Geometry check sheet. Reference: the model listing, model coordinates, mm. Face numbers are marked on the shaded views. A direction names the side the tool comes from. Coordinates: 2 decimals unless noted, no trailing zeros. Write each loop counter-clockwise with the first axis right and the second up, starting at its lowest first coordinate (ties: lowest second). Pieces come first, ordered by that corner, then holes. Notation, with made-up numbers: (59, 48) -> (67, 48) arc R15 cw to (67, 61) -> close; hole circle Ø5 at (52, 38.25). An arc over 180 degrees is marked (long way). Use a Markdown table: item, result.
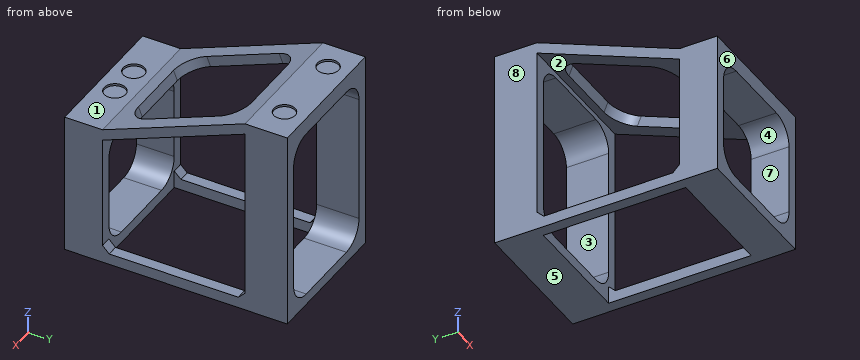
```python
from build123d import *

# Parameters (mm, degrees)
BOSS_EXTRUDE1_DEPTH = 58.71
SKETCH4_R           = 4.8
CUT_EXTRUDE1_DEPTH  = 1
SKETCH5_R           = 4.8
CUT_EXTRUDE2_DEPTH  = 1
SKETCH6_W           = 19
SKETCH6_H           = 26
BOSS_EXTRUDE3_DEPTH = 58.71
SKETCH7_W           = 58.71
SKETCH7_H           = 17
SKETCH7_H_2         = 19
BOSS_EXTRUDE4_DEPTH = 59
BOSS_EXTRUDE5_DEPTH = 3
CUT_EXTRUDE3_DEPTH  = 17
CUT_EXTRUDE4_START  = -19
CUT_EXTRUDE4_DEPTH  = 19
CUT_EXTRUDE5_DEPTH  = 4.632332886
SKETCH12_W          = 5
SKETCH12_H          = 5
BOSS_EXTRUDE6_DEPTH = 100
CHAMFER1_SIZE       = 3


with BuildPart() as part:
    # Sketch3 → Boss-Extrude1 (new body)
    with BuildSketch(Plane.YZ):
        Polygon((0, 5), (0, 0), (17, 0), (81, 26), (100, 26), (100, 31), (81, 31), (17, 5), align=None)
    extrude(amount=BOSS_EXTRUDE1_DEPTH)

    # Sketch4 → Cut-Extrude1 (cut)
    with BuildSketch(Plane.XY.offset(31)):
        with Locations((12.75, 90.5)):
            Circle(SKETCH4_R)
        with Locations((47.2, 90.5)):
            Circle(SKETCH4_R)
    extrude(amount=-CUT_EXTRUDE1_DEPTH, mode=Mode.SUBTRACT)

    # Sketch5 → Cut-Extrude2 (cut)
    with BuildSketch(Plane.XY.offset(5)):
        with Locations((21.94, 8.5)):
            Circle(SKETCH5_R)
        with Locations((36.94, 8.5)):
            Circle(SKETCH5_R)
    extrude(amount=-CUT_EXTRUDE2_DEPTH, mode=Mode.SUBTRACT)

    # Sketch6 → Boss-Extrude3 (add)
    with BuildSketch(Plane.YZ.offset(58.71)):
        with Locations((90.5, 13)):
            Rectangle(SKETCH6_W, SKETCH6_H)
    extrude(amount=-BOSS_EXTRUDE3_DEPTH)

    # Sketch7 → Boss-Extrude4 (add)
    with BuildSketch(Plane(origin=(0, 0, 0), x_dir=(1, 0, 0), z_dir=(0, 0, -1))):
        with Locations((29.355, -8.5)):
            Rectangle(SKETCH7_W, SKETCH7_H)
        with Locations((29.355, -90.5)):
            Rectangle(SKETCH7_W, SKETCH7_H_2)
    extrude(amount=BOSS_EXTRUDE4_DEPTH)

    # Sketch8 → Boss-Extrude5 (add)
    with BuildSketch(Plane.YZ.offset(58.71)):
        Polygon((100, 31), (81, 31), (17, 5), (0, 5), (0, -59), (17, -59), (17, 0), (81, 26), (81, -59), (100, -59), align=None)
    extrude(amount=BOSS_EXTRUDE5_DEPTH)

    # Sketch9 → Cut-Extrude3 (cut)
    with BuildSketch(Plane.XZ):
        with BuildLine():
            Line((15, -2.5), (46.71, -2.5))
            ThreePointArc((46.71, -2.5), (53.781067812, -5.428932188), (56.71, -12.5))
            Line((56.71, -12.5), (56.71, -44))
            ThreePointArc((56.71, -44), (53.781067812, -51.071067812), (46.71, -54))
            Line((46.71, -54), (15, -54))
            ThreePointArc((15, -54), (7.928932188, -51.071067812), (5, -44))
            Line((5, -44), (5, -12.5))
            ThreePointArc((5, -12.5), (7.928932188, -5.428932188), (15, -2.5))
        make_face()
    extrude(amount=-CUT_EXTRUDE3_DEPTH, mode=Mode.SUBTRACT)

    # Sketch10 → Cut-Extrude4 (cut)
    with BuildSketch(Plane(origin=(0, 100, 0), x_dir=(-1, 0, 0), z_dir=(0, 1, 0)).offset(CUT_EXTRUDE4_START)):
        with BuildLine():
            Line((-46.71, 23.5), (-15, 23.5))
            ThreePointArc((-15, 23.5), (-7.928932188, 20.571067812), (-5, 13.5))
            Line((-5, 13.5), (-5, -44))
            ThreePointArc((-5, -44), (-7.928932188, -51.071067812), (-15, -54))
            Line((-15, -54), (-46.71, -54))
            ThreePointArc((-46.71, -54), (-53.781067812, -51.071067812), (-56.71, -44))
            Line((-56.71, -44), (-56.71, 13.5))
            ThreePointArc((-56.71, 13.5), (-53.781067812, 20.571067812), (-46.71, 23.5))
        make_face()
    extrude(amount=CUT_EXTRUDE4_DEPTH, mode=Mode.SUBTRACT)

    # Sketch11 → Cut-Extrude5 (cut)
    with BuildSketch(Plane(origin=(0, 0.664710813, -1.636211232), x_dir=(1, 0, 0), z_dir=(0, -0.376377046955938, 0.9264665771223093))):
        with BuildLine():
            Line((17, 79.711481203), (44.71, 79.711481203))
            ThreePointArc((44.71, 79.711481203), (51.781067812, 76.782549014), (54.71, 69.711481203))
            Line((54.71, 69.711481203), (54.71, 34.631817046))
            ThreePointArc((54.71, 34.631817046), (51.781067812, 27.560749234), (44.71, 24.631817046))
            Line((44.71, 24.631817046), (17, 24.631817046))
            ThreePointArc((17, 24.631817046), (9.928932188, 27.560749234), (7, 34.631817046))
            Line((7, 34.631817046), (7, 69.711481203))
            ThreePointArc((7, 69.711481203), (9.928932188, 76.782549014), (17, 79.711481203))
        make_face()
    extrude(amount=-CUT_EXTRUDE5_DEPTH, mode=Mode.SUBTRACT)

    # Sketch12 → Boss-Extrude6 (add)
    with BuildSketch(Plane.XZ):
        with Locations((2.5, -56.5)):
            Rectangle(SKETCH12_W, SKETCH12_H)
        with Locations((59.21, -56.5)):
            Rectangle(SKETCH12_W, SKETCH12_H)
    extrude(amount=-BOSS_EXTRUDE6_DEPTH)

    # Chamfer1
    chamfer1_edges = [part.edges().sort_by_distance(p)[0] for p in [
        (2.5, 17, -54),
        (2.5, 81, -54),
        (59.21, 81, -54),
        (59.21, 17, -54),
    ]]
    chamfer(chamfer1_edges, length=CHAMFER1_SIZE)


solid = part.part
```
Item 1: Depth check by flat-ended pin: P1, Ø12, axis at x = 27.5, y = 19, coming from the +Z side; P2, Ø13.5, axis at x = 37.5, y = 5, coming from the +Z side; P3, Ø3, axis at x = 7, y = 56, coming from the -Z side. Enter the tip coordinate at first touch or a pass-through.
Answer block:
| item | result |
|---|---|
| P1 | stops at z = 7.63 |
| P2 | stops at z = 5 |
| P3 | stops at z = 15.23 |
Item 2: Section check A-A on x = 36.94. Record the boundary of the cut face in (y, z).
Answer block:
| item | result |
|---|---|
| outline | (0, -59) -> (17, -59) -> (17, -54) -> (0, -54) -> close; (0, -2.5) -> (17, -2.5) -> (17, 0) -> (25.23, 3.34) -> (23.49, 7.63) -> (17, 5) -> (13.3, 5) -> (13.3, 4) -> (3.7, 4) -> (3.7, 5) -> (0, 5) -> close; (74.51, 28.37) -> (76.26, 24.07) -> (81, 26) -> (81, 23.5) -> (100, 23.5) -> (100, 31) -> (81, 31) -> close; (81, -59) -> (100, -59) -> (100, -54) -> (81, -54) -> close |
Item 3: Section check C-C on y = 8.5. Record the boundary of the cut face in (x, z), then the cut area to 3 significant figures.
Answer block:
| item | result |
|---|---|
| outline | (0, -59) -> (61.71, -59) -> (61.71, 5) -> (41.74, 5) -> (41.74, 4) -> (32.14, 4) -> (32.14, 5) -> (26.74, 5) -> (26.74, 4) -> (17.14, 4) -> (17.14, 5) -> (0, 5) -> close; hole (5, -44) arc R10 ccw to (15, -54) -> (46.71, -54) arc R10 ccw to (56.71, -44) -> (56.71, -12.5) arc R10 ccw to (46.71, -2.5) -> (15, -2.5) arc R10 ccw to (5, -12.5) -> close |
| area | 1,350 mm^2 |
Item 4: Tool access check on the marked faces 1, 2, 3, 4 and 5. Record the directions out of +Z, -Z, +X, -X, +Y, -Y that give a thin tool (end or side, any length) a straight path to the whole face; none if there is none.
Answer block:
| item | result |
|---|---|
| face 1 | +Z, +X, -X, -Y |
| face 2 | +X, -X |
| face 3 | +Y |
| face 4 | +Y, -Y |
| face 5 | -Z, +X, -X, +Y, -Y |
Item 5: Thickness scan on L1, parallel to X at y = 95, z = -15.5; L2, parallel to Z at x = 43.5, y = 4; L3, parallel to Z at x = 30.5, y = 88.5. Record the ranges inside material, lowest first. Write a range as [from, to].
Answer block:
| item | result |
|---|---|
| L1 | x = [0, 5], [56.71, 61.71] |
| L2 | z = [-59, -54], [-2.5, 5] |
| L3 | z = [-59, -54], [23.5, 31] |
Item 6: Section check D-D on z = 18.5. Record the boundary of the cut face in (x, y).
Answer block:
| item | result |
|---|---|
| outline | (0, 50.23) -> (7, 50.23) -> (7, 62.54) -> (0, 62.54) -> close; (0, 81) -> (6.34, 81) -> (6.34, 100) -> (0, 100) -> close; (54.71, 50.23) -> (61.71, 50.23) -> (61.71, 62.54) -> (54.71, 62.54) -> close; (55.37, 81) -> (61.71, 81) -> (61.71, 100) -> (55.37, 100) -> close |
Item 7: Section check B-B on z = -40. Record the boundary of the cut face in (x, y), then the cut area to 3 significant figures.
Answer block:
| item | result |
|---|---|
| outline | (0, 0) -> (5, 0) -> (5, 17) -> (0, 17) -> close; (0, 81) -> (5, 81) -> (5, 100) -> (0, 100) -> close; (56.71, 0) -> (61.71, 0) -> (61.71, 17) -> (56.71, 17) -> close; (56.71, 81) -> (61.71, 81) -> (61.71, 100) -> (56.71, 100) -> close |
| area | 360 mm^2 |
Item 8: Mould release check, pull along X, two halves, no side actions. Record for the marked faces 6, 7 and 8: +X half, -X half, draft (parallel to the pull), parting line (faces both ways), or undercut.
Answer block:
| item | result |
|---|---|
| face 6 | draft |
| face 7 | undercut |
| face 8 | -X half |
